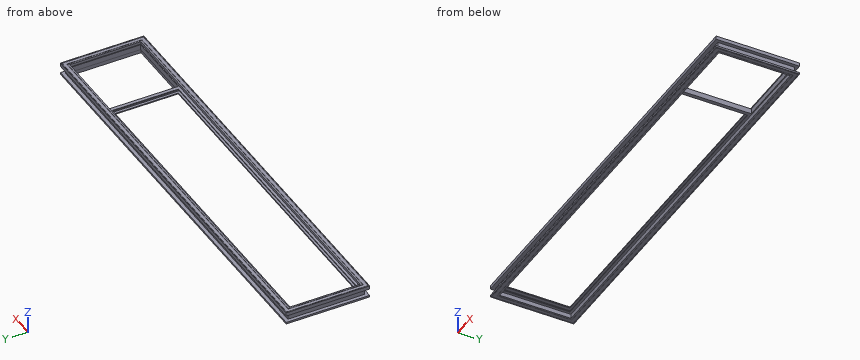
```python
from build123d import *

# Parameters (mm, degrees)
CUT_EXTRUDE1_START  = -19.05
SKETCH3_W           = 254
SKETCH3_H           = 254
CUT_EXTRUDE1_DEPTH  = 19.05
BOSS_EXTRUDE1_DEPTH = 266.7
SKETCH7_W           = 12.7
SKETCH7_H           = 3.175


with BuildPart() as part:
    # Sweep1: sweep along a path in Sketch2
    with BuildLine(Plane.XY) as sweep1_path:
        Line((762, 152.4), (-762, 152.4))
        Line((-762, 152.4), (-762, -152.4))
        Line((-762, -152.4), (762, -152.4))
        Line((762, -152.4), (762, 152.4))
    # Sketch1 → Sweep1 (sweep)
    with BuildSketch(Plane(origin=(0, 0, 0), x_dir=(1, 0, 0), z_dir=(0, 1, 0))):
        with BuildLine():
            Line((-762, -25.4), (-759.587, -25.4))
            ThreePointArc((-759.587, -25.4), (-758.825, -24.638), (-758.063, -25.4))
            Line((-758.063, -25.4), (-746.887, -25.4))
            ThreePointArc((-746.887, -25.4), (-746.125, -24.638), (-745.363, -25.4))
            Line((-745.363, -25.4), (-739.775, -25.4))
            Line((-739.775, -25.4), (-739.775, -15.875))
            Line((-739.775, -15.875), (-730.25, -15.875))
            Line((-730.25, -15.875), (-730.25, -12.7))
            Line((-730.25, -12.7), (-742.95, -12.7))
            Line((-742.95, -12.7), (-742.95, 0))
            Line((-742.95, 0), (-730.25, 0))
            Line((-730.25, 0), (-730.25, 3.175))
            Line((-730.25, 3.175), (-739.775, 3.175))
            Line((-739.775, 3.175), (-739.775, 19.05))
            Line((-739.775, 19.05), (-745.744, 19.05))
            ThreePointArc((-745.744, 19.05), (-746.125, 18.669), (-746.506, 19.05))
            Line((-746.506, 19.05), (-758.444, 19.05))
            ThreePointArc((-758.444, 19.05), (-758.825, 18.669), (-759.206, 19.05))
            Line((-759.206, 19.05), (-762, 19.05))
            Line((-762, 19.05), (-762, 12.7))
            Line((-762, 12.7), (-749.3, 12.7))
            Line((-749.3, 12.7), (-749.3, -12.7))
            Line((-749.3, -12.7), (-762, -12.7))
            Line((-762, -12.7), (-762, -25.4))
        make_face()
    sweep(path=sweep1_path.line, transition=Transition.RIGHT)

    # Sketch3 → Cut-Extrude1 (cut)
    with BuildSketch(Plane.XY.offset(15.875).offset(CUT_EXTRUDE1_START)):
        with Locations((609.6, 0)):
            Rectangle(SKETCH3_W, SKETCH3_H)
    extrude(amount=CUT_EXTRUDE1_DEPTH, mode=Mode.SUBTRACT)

    # Sketch6 → Boss-Extrude1 (add)
    with BuildSketch(Plane(origin=(0, -133.35, 0), x_dir=(1, 0, 0), z_dir=(0, 1, 0))):
        Polygon((482.6, 3.175), (482.6, -15.875), (469.9, -15.875), (469.9, -12.7), (479.425, -12.7), (479.425, 0), (469.9, 0), (469.9, 3.175), align=None)
    extrude(amount=BOSS_EXTRUDE1_DEPTH)

    # Sweep2: sweep along a path in Sketch8
    with BuildLine(Plane(origin=(0, 0, -3.175), x_dir=(-1, 0, 0), z_dir=(0, 0, -1))) as sweep2_path:
        Line((-482.6, -127), (-736.6, -127))
        Line((-736.6, -127), (-736.6, 127))
        Line((-736.6, 127), (-482.6, 127))
    # Sketch7 → Sweep2 (sweep)
    with BuildSketch(Plane(origin=(482.6, 0, 0), x_dir=(0, 0, -1), z_dir=(1, 0, 0))):
        with Locations((-6.35, -128.5875)):
            Rectangle(SKETCH7_W, SKETCH7_H)
    sweep(path=sweep2_path.line, transition=Transition.RIGHT)


solid = part.part
```
CAD build for the part. Positions are in the model's coordinates, mm. Give positions to 0.01 mm unless a question says otherwise; leave off trailing zeros. Write each question's results on one line, items separated by ' | '.
1. Drop flat-ended pins along their axis: P1, Ø8, axis at x = 44.5, z = 5, coming from the -Y side; P2, Ø8, axis at y = -57, z = 0.5, coming from the +X side; P3, Ø20.5, axis at y = -43.5, z = 0.5, coming from the -X side. Give the stop position or say it passes through.
Geometry check:
P1: y = -139.7 | P2: x = 749.3 | P3: x = -749.3
2. Cut at A-A, the plane x = 580. Give the number of separate pieces and of enclosed holes in the cut face, then the cut area to 3 significant figures.
Geometry check:
separate pieces: 2 | enclosed holes: 2 | area: 1,370 mm²
3. Wall check: probe 1 along X at (y, z) = (85.5, 13.5); probe 2 along X at (y, z) = (45, 2.5) (3 decimals); probe 3 along X at (y, z) = (19, -1). Give the ranges that are in metal, low to high. Write a range as [from, to].
Geometry check:
probe 1: [-762, -730.25], [469.9, 482.6], [736.6, 762] | probe 2: [-749.3, -742.95], [479.425, 482.6], [736.6, 739.775], [742.95, 749.3] | probe 3: [-749.3, -730.25], [469.9, 482.6], [736.6, 749.3]
